```python
from build123d import *

# Parameters (mm, degrees)
F0_R     = 12
F0_R_2   = 5
F1_DEPTH = 7
F0_R_3   = 12.75
F2_DEPTH = 2.75
F3_R     = 17
F3_R_2   = 5
F4_DEPTH = 6
F5_SIZE  = 1.5
F6_R     = 17
F6_R_2   = 12
F6_R_3   = 5
F7_DEPTH = 6
F8_SIZE  = 1.5


with BuildPart() as f1:
    # F0 (on Front) → F1 (new body, symmetric)
    with BuildSketch(Plane.XZ):
        with Locations((-137.7102136612, -19.4580089301)):
            Circle(F0_R)
        with Locations((-137.7102136612, -19.4580089301)):
            Circle(F0_R_2, mode=Mode.SUBTRACT)
    extrude(amount=F1_DEPTH, both=True)

    # F0 (on Front) → F2 (join, symmetric)
    with BuildSketch(Plane.XZ):
        with Locations((-137.7102136612, -19.4580089301)):
            Circle(F0_R_3)
        with Locations((-137.7102136612, -19.4580089301)):
            Circle(F0_R, mode=Mode.SUBTRACT)
    extrude(amount=F2_DEPTH, both=True)

    # F3 (on face) → F4 (join)
    with BuildSketch(Plane.XZ.offset(7)):
        with Locations((-137.7102136612, -19.4580089301)):
            Circle(F3_R)
        with Locations((-137.7102136612, -19.4580089301)):
            Circle(F3_R_2, mode=Mode.SUBTRACT)
    extrude(amount=F4_DEPTH)

    # F5
    f5_edges = [f1.edges().sort_by_distance(p)[0] for p in [
        (-154.710214, -7, -19.458009),
    ]]
    chamfer(f5_edges, length=F5_SIZE)

    # F6 (on face) → F7 (join)
    with BuildSketch(Plane(origin=(0, 7, 0), x_dir=(-1, 0, 0), z_dir=(0, 1, 0))):
        with Locations((137.7102136612, -19.4580089301)):
            Circle(F6_R)
        with Locations((137.7102136612, -19.4580089301)):
            Circle(F6_R_2, mode=Mode.SUBTRACT)
        with Locations((137.7102136612, -19.4580089301)):
            Circle(F6_R_2)
        with Locations((137.7102136612, -19.4580089301)):
            Circle(F6_R_3, mode=Mode.SUBTRACT)
    extrude(amount=F7_DEPTH)

    # F8
    f8_edges = [f1.edges().sort_by_distance(p)[0] for p in [
        (-120.710214, 7, -19.458009),
    ]]
    chamfer(f8_edges, length=F8_SIZE)


solid = f1.part
```
Can you work these out from the model? Positions are in its coordinate system, mm. A direction names the side the tool comes from. Round coordinates to 2 decimals unless told otherwise and drop trailing zeros. Loops run counter-clockwise (first coordinate to the right, second up) from the corner with the lowest first, then second, coordinate; pieces in that order, holes last.
Item 1: Which directions (+Z, -Z, +X, -X, +Y, -Y) give clear straight access to the entire face, cutting with the end or side of a thin tool? Please do faces 4 (the flat face through (-142, -13, -23)), 5 (the cylindrical face through (-126.264, -4.905, -15.854)).
Item 2: Suppose I cut it at A-A, the plane y = 9. Write out the boundary of the cut face in (x, z).
Item 3: Suppose I cut it at B-B, the plane y = -7.5. Write out the boundary of the cut face in (x, z).
Item 4: If we mould it in two halves opening along Y, with no side actions, what happens to faces 1 (the flat face through (-133.7, 13, -23)), 2 (the cylindrical face through (-153.925, 10.718, -14.352)), 3 (the flat face through (-146, 7, -29))? For each: +Y half, -Y half, draft (parallel to the pull), parting line (faces both ways), or undercut.
Item 5: Will these pins go through, and if not, where does the flat tip stop? pin 1 Ø2 at (y, z) = (-9, -17) entering from +X; pin 2 Ø10 at (y, z) = (7, -27) entering from -X; pin 3 Ø2 at (y, z) = (-5.5, -15.5) entering from +X; pin 4 Ø5 at (x, z) = (-138, -19) entering from -Y.
Item 6: Please list where these lines run through material, in increasing order: L1, parallel to Y at x = -148.5, z = -25.5; L2, parallel to Y at x = -152, z = -16.5; L3, parallel to Z at x = -135, y = -4.5.
Reported:
1. face 4: +Z, -Z, +X, -X, -Y
1. face 5: none
2. outline: circle Ø34 at (-137.71, -19.46); hole circle Ø10 at (-137.71, -19.46)
3. outline: circle Ø32 at (-137.71, -19.46); hole circle Ø10 at (-137.71, -19.46)
4. face 1: +Y half
4. face 2: draft
4. face 3: undercut
5. pin 1: stops at x = -120.77
5. pin 2: stops at x = -154.48
5. pin 3: stops at x = -126.08
5. pin 4: passes through
6. L1: y = -13 to -7, -2.75 to 2.75, 7 to 13
6. L2: y = -13 to -7, 7 to 13
6. L3: z = -31.15 to -23.66, -15.26 to -7.77
